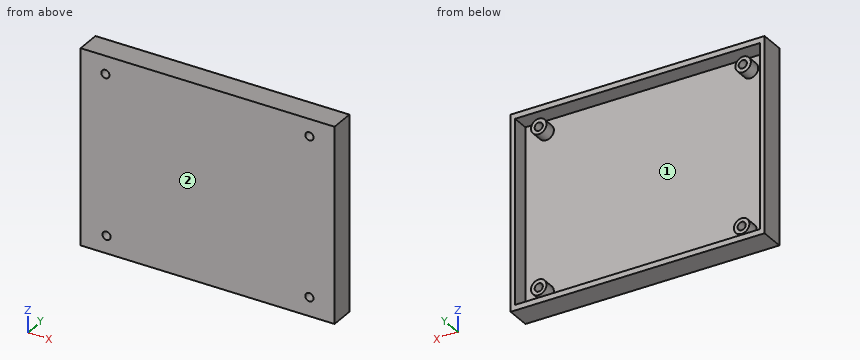
```python
from build123d import *

# Parameters (mm, degrees)
SKETCH1_W           = 101.6
SKETCH1_H           = 76.2
SKETCH1_R           = 3.201261119
BOSS_EXTRUDE4_DEPTH = 3
SKETCH1_8_W         = 105.264465986
SKETCH1_8_H         = 80.768961322
SKETCH1_8_W_2       = 101.6
SKETCH1_8_H_2       = 76.2
BOSS_EXTRUDE6_DEPTH = 10
SKETCH1_10_R        = 3.201261119
SKETCH1_10_R_2      = 1.7
BOSS_EXTRUDE7_DEPTH = 8


with BuildPart() as part:
    # Sketch1 → Boss-Extrude4 (new body)
    with BuildSketch(Plane(origin=(0, 0, 0), x_dir=(1, 0, 0), z_dir=(0, 1, 0))):
        Rectangle(SKETCH1_W, SKETCH1_H)
        with Locations(Location((42.20618594, -33.358721943, 0), (0, 0, 270))):
            Circle(SKETCH1_R, mode=Mode.SUBTRACT)
        with Locations(Location((-42.51175292, -32.859842277, 0), (0, 0, 270))):
            Circle(SKETCH1_R, mode=Mode.SUBTRACT)
        with Locations(Location((42.225895984, 32.494174618, 0), (0, 0, 270))):
            Circle(SKETCH1_R, mode=Mode.SUBTRACT)
        with Locations(Location((-41.91, 33.147, 0), (0, 0, 270))):
            Circle(SKETCH1_R, mode=Mode.SUBTRACT)
    extrude(amount=BOSS_EXTRUDE4_DEPTH)

    # Sketch1_8 → Boss-Extrude6 (add)
    with BuildSketch(Plane(origin=(0, 0, 0), x_dir=(1, 0, 0), z_dir=(0, 1, 0))):
        Rectangle(SKETCH1_8_W, SKETCH1_8_H)
        Rectangle(SKETCH1_8_W_2, SKETCH1_8_H_2, mode=Mode.SUBTRACT)
    extrude(amount=BOSS_EXTRUDE6_DEPTH)

    # Sketch1_10 → Boss-Extrude7 (add)
    # profile 1 of 4: a face of its own
    with BuildSketch(Plane(origin=(0, 0, 0), x_dir=(1, 0, 0), z_dir=(0, 1, 0))):
        with Locations(Location((-41.91, 33.147, 0), (0, 0, 270))):
            Circle(SKETCH1_10_R)
        with Locations(Location((-41.91, 33.147, 0), (0, 0, 270))):
            Circle(SKETCH1_10_R_2, mode=Mode.SUBTRACT)
    # profile 2 of 4: a face of its own
    with BuildSketch(Plane(origin=(0, 0, 0), x_dir=(1, 0, 0), z_dir=(0, 1, 0))):
        with Locations(Location((42.20618594, -33.358721943, 0), (0, 0, 270))):
            Circle(SKETCH1_10_R)
        with Locations(Location((42.205092494, -33.267543495, 0), (0, 0, 270))):
            Circle(SKETCH1_10_R_2, mode=Mode.SUBTRACT)
    # profile 3 of 4: a face of its own
    with BuildSketch(Plane(origin=(0, 0, 0), x_dir=(1, 0, 0), z_dir=(0, 1, 0))):
        with Locations(Location((-42.51175292, -32.859842277, 0), (0, 0, 270))):
            Circle(SKETCH1_10_R)
        with Locations(Location((-42.370602661, -32.936523162, 0), (0, 0, 270))):
            Circle(SKETCH1_10_R_2, mode=Mode.SUBTRACT)
    # profile 4 of 4: a face of its own
    with BuildSketch(Plane(origin=(0, 0, 0), x_dir=(1, 0, 0), z_dir=(0, 1, 0))):
        with Locations(Location((42.225895984, 32.494174618, 0), (0, 0, 270))):
            Circle(SKETCH1_10_R)
        with Locations(Location((42.205092494, 32.605502829, 0), (0, 0, 270))):
            Circle(SKETCH1_10_R_2, mode=Mode.SUBTRACT)
    extrude(amount=BOSS_EXTRUDE7_DEPTH)


solid = part.part
```
For this review, take the finished solid that the model builds, in its own axes (mm). Face numbers are marked on the shaded views. Give positions to 0.01 mm unless a question says otherwise; leave off trailing zeros. Write each loop counter-clockwise with the first axis right and the second up, starting at its lowest first coordinate (ties: lowest second). Pieces come first, ordered by that corner, then holes. Notation, with made-up numbers: M 78,-7 L 91,-7 A9 cw 91,6 Z; hole C 33,13.25 d9. An arc over 180 degrees is marked long. Answer as a JSON object with one key per item and string values. Group by question number.
Item 1: Consider section B-B on z = -2.5. Write out the cut boundary in (x, y).
Item 2: Draft analysis for pull direction X (two halves, no side actions). For the marked faces 1 and 2, state which applies: +X half, -X half, draft (parallel to the pull), parting line (faces both ways), or undercut.
Item 3: For probe 1 along Z at (x, y) = (-9, 4.25); probe 2 along X at (y, z) = (8, 8.5); probe 3 along Y at (x, z) = (36.5, 13), list the stretches that pass through material, from the lowest coordinate up. Write a range as [from, to].
Item 4: For pin 1 Ø6 at (x, z) = (-41, -28.5) entering from +Y; pin 2 Ø3 at (x, z) = (42.21, 33.27) entering from +Y; pin 3 Ø1.5 at (x, z) = (29, -2) entering from +Y, all flat-tipped, find the tip position at first contact; note any pin that passes through.
Item 5: Consider section A-A on y = 6.75. Count the separate pieces of the cut face and the enclosed holes in it, plus the area to 3 significant figures.
Item 6: Consider section C-C on x = -32.5. Write out the cut boundary in (y, z).
Check result:
{
 "1": {"outline": "M -52.63,0 L 52.63,0 L 52.63,10 L 50.8,10 L 50.8,3 L -50.8,3 L -50.8,10 L -52.63,10 Z"},
 "2": {"face 1": "undercut", "face 2": "draft"},
 "3": {"probe 1": "z = [-40.38, -38.1], [38.1, 40.38]", "probe 2": "x = [-52.63, -50.8], [50.8, 52.63]", "probe 3": "y = [0, 3]"},
 "4": {"pin 1": "stops at y = 8", "pin 2": "passes through", "pin 3": "stops at y = 3"},
 "5": {"separate pieces": "5", "enclosed holes": "5", "area": "853 mm^2"},
 "6": {"outline": "M 0,-40.38 L 10,-40.38 L 10,-38.1 L 3,-38.1 L 3,38.1 L 10,38.1 L 10,40.38 L 0,40.38 Z"}
}
